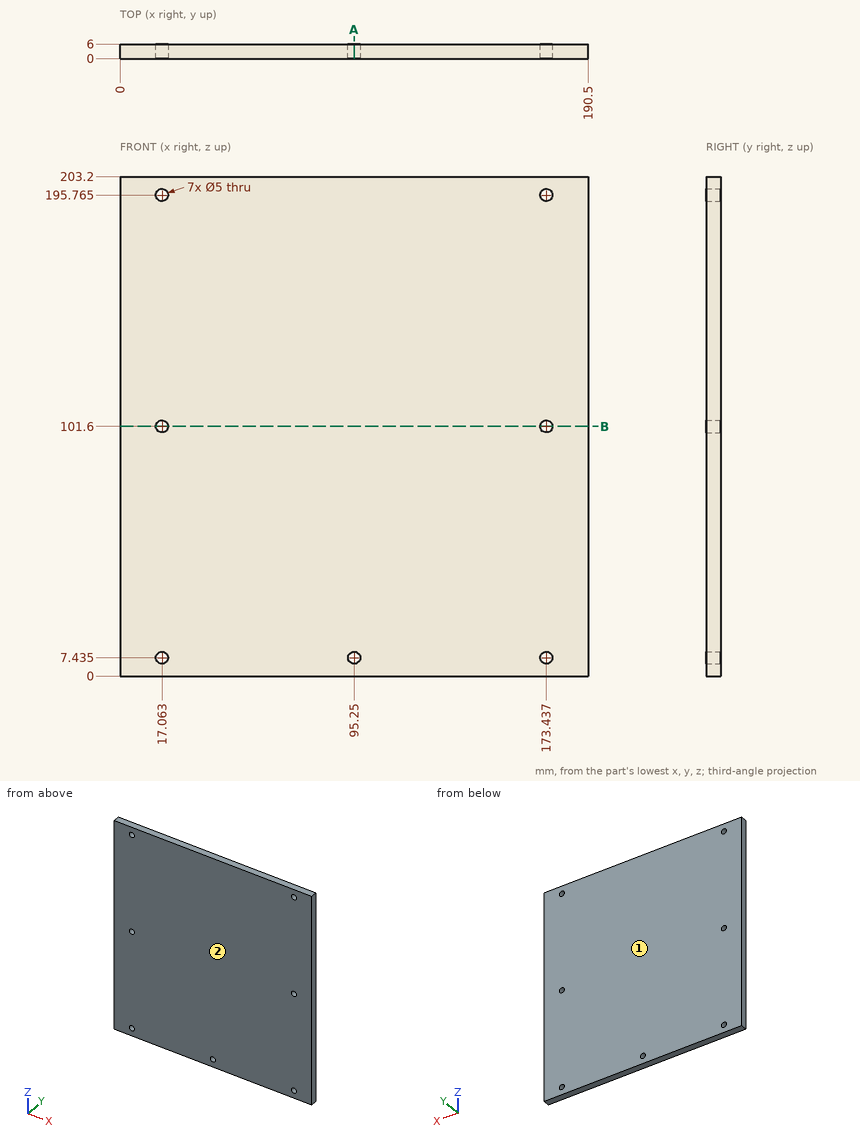
Print and shaded views of the part. All mm, measured from the part's lowest x, y and z. Coordinates: 2 decimals unless noted, no trailing zeros. Order: outer loops, then holes, each group sorted by start corner. A loop starts at its lowest first (then second) coordinate and runs counter-clockwise, first axis right, second up. Notation, with made-up numbers: M -17,10 L -5,10 A15 ccw -5,35 Z; hole C 15.5,-38.5 d9. An arc over 180 degrees is marked long. Answer as CSV lines item,"result".
1) Drill centre lines: L1, parallel to X at y = 3.8, z = 101.6; L2, parallel to X at y = 4, z = 99.5; L3, parallel to Z at x = 94, y = 5.1. Where is each one in solid material? Low to high. Write a range as from..to.
Verdict:
L1,"0..14.56, 19.56..170.94, 175.94..190.5"
L2,"0..15.71, 18.42..172.08, 174.79..190.5"
L3,"0..5.27, 9.6..203.2"
2) Mould opens along Y. For the marked faces 1 and 2 say: released by +Y, released by -Y, zero draft, split by the parting line, or undercut.
Verdict:
face 1,"released by +Y"
face 2,"released by -Y"
3) Cut at A-A (x = 95.25). List the corners of the cut face in (y, z) (3 decimals), then the cut area to 3 significant figures.
Verdict:
outline,"M 0,0 L 6,0 L 6,4.935 L 0,4.935 Z; M 0,9.935 L 6,9.935 L 6,203.2 L 0,203.2 Z"
area,"1,190 mm2"
4) Cut at B-B (z = 101.6). List the corners of the cut face in (x, y), then the cut area to 3 significant figures.
Verdict:
outline,"M 0,0 L 14.56,0 L 14.56,6 L 0,6 Z; M 19.56,0 L 170.94,0 L 170.94,6 L 19.56,6 Z; M 175.94,0 L 190.5,0 L 190.5,6 L 175.94,6 Z"
area,"1,080 mm2"
5) Flat gauge pin, fed straight in: P1, Ø3, axis at x = 17.06, z = 101.6, coming from the +Y side. Where does the tip first touch, or does it go through?
Verdict:
P1,"through"
